Geometry check sheet. Reference: the model listing, model coordinates, mm. Give positions to 0.01 mm unless a question says otherwise; leave off trailing zeros. Loops run counter-clockwise (first coordinate to the right, second up) from the corner with the lowest first, then second, coordinate; pieces in that order, holes last. Notation, with made-up numbers: (-24.75, 66) - (16.25, 66) arc R20 cw to (16.25, 77) - close; hole circle Ø7 at (-14.5, -37.75). An arc over 180 degrees is marked (long way). Use a Markdown table: item, result. Add a question column.
1. Draft check along Y on faces 1 (the cylindrical face through (5.48, 1.67, -0.53)), 2 (the flat face through (0, -1, -1)), 3 (the conical face through (2.34, -0.02, 0.07)). Enter one of: pulls with the +Y half, pulls with the -Y half, needs draft (parallel to the pull), parting line crosses it, or undercut.
2. Cross-section at A-A on x = 1. Enter the section's corners in (y, z).
3. Material ranges on L1, parallel to Y at x = 0.5, z = 0.75; L2, parallel to X at y = -0.5, z = -2; L3, parallel to X at y = 3, z = 0, recorded low to high.
4. Cross-section at B-B on x = 5.75. Enter the section's corners in (y, z).
5. Depth check by flat-ended pin: P1, Ø1, axis at x = 7, z = 0.5, coming from the -Y side; P2, Ø1.5, axis at x = 6, z = -2, coming from the +Y side; P3, Ø1.5, axis at y = 2, z = 2.5, coming from the +X side. Enter the tip coordinate at first touch or a pass-through.
Autodesk Inventor part; units mm, degrees
ref_plane "Work Plane1" through (66.6877, 0, 0) normal (0, 0, -1) x (1, 0, 0)
ref_plane "YZ Plane" through (0, 0, 0) normal (1, 0, 0) x (0, 1, 0)
ref_plane "XZ Plane" through (0, 0, 0) normal (0, 1, 0) x (-1, 0, 0)
sketch "Sketch1" plane through (0, 0, 0) normal (0, 0, 1) x (1, 0, 0)
  line L0 (9.525, 0) -> (9.525, 1.7526)
  line L1 (9.525, 1.7526) -> (2.4638, 1.7526)
  line L2 (0, 3.3401) -> (0, 1.2192)
  line L3 (0, 1.2192) -> (1.6764, 1.2192)
  line L4 (1.6764, 1.2192) -> (2.3803, 0)
  line L5 (2.3803, 0) -> (9.525, 0)
  line L6 (0, 3.3401) -> (0.6376, 3.3401)
  line L7 (0.6376, 3.3401) -> (2.4638, 1.7526)
  line L8 (-1.905, 0) -> (11.43, 0)
  line L9 (0, -0.668) -> (0, 4.0081)
  dimension "d0" = 9.525
  dimension "d1" = 1.6764
  dimension "d2" = 3.5052
  dimension "d3" = 2.4638
  dimension "d4" = 41
  dimension "d5" = 2.4384
  dimension "d6" = 60
  dimension "d7" = 6.6802
revolve "Body" add sketch "Sketch1" angle 360 about axis through (2.3803, 0, 0) along (1, 0, 0) contours L5 L4 L3 L2 L6 L7 L1 L0
sketch "Sketch2" plane through (0, 0, 0) normal (-1, 0, 0) x (0, 0, 1)
  circle A0 centre (0, 0) radius 3.3401
  circle A1 centre (0, 0) radius 1.2192
  line L0 (0.9421, 0.2524) -> (1.1777, 0.3156)
  line L1 (0.9421, -0.2524) -> (1.1777, -0.3156)
  arc A2 (0.9421, -0.2524) -> (0.9421, 0.2524) centre (0, 0) ccw
  arc A3 (1.1777, -0.3156) -> (1.1777, 0.3156) centre (0, 0) ccw
  line L2 (0, -4.6761) -> (0, 4.6761)
  line L3 (-4.6761, 0) -> (4.6761, 0)
  line L4 (0.9421, 0.2524) -> (0, 0) construction
  line L5 (0, 0) -> (0.9421, -0.2524) construction
  line L6 (0.2524, 0.9421) -> (0.3156, 1.1777)
  line L7 (0.6897, 0.6897) -> (0.8621, 0.8621)
  arc A4 (0.6897, 0.6897) -> (0.2524, 0.9421) centre (0, 0) ccw
  arc A5 (0.8621, 0.8621) -> (0.3156, 1.1777) centre (0, 0) ccw
  line L8 (-0.6897, 0.6897) -> (-0.8621, 0.8621)
  line L9 (-0.2524, 0.9421) -> (-0.3156, 1.1777)
  arc A6 (-0.2524, 0.9421) -> (-0.6897, 0.6897) centre (0, 0) ccw
  arc A7 (-0.3156, 1.1777) -> (-0.8621, 0.8621) centre (0, 0) ccw
  line L10 (-0.9421, -0.2524) -> (-1.1777, -0.3156)
  line L11 (-0.9421, 0.2524) -> (-1.1777, 0.3156)
  arc A8 (-0.9421, 0.2524) -> (-0.9421, -0.2524) centre (0, 0) ccw
  arc A9 (-1.1777, 0.3156) -> (-1.1777, -0.3156) centre (0, 0) ccw
  line L12 (-0.2524, -0.9421) -> (-0.3156, -1.1777)
  line L13 (-0.6897, -0.6897) -> (-0.8621, -0.8621)
  arc A10 (-0.6897, -0.6897) -> (-0.2524, -0.9421) centre (0, 0) ccw
  arc A11 (-0.8621, -0.8621) -> (-0.3156, -1.1777) centre (0, 0) ccw
  line L14 (0.6897, -0.6897) -> (0.8621, -0.8621)
  line L15 (0.2524, -0.9421) -> (0.3156, -1.1777)
  arc A12 (0.2524, -0.9421) -> (0.6897, -0.6897) centre (0, 0) ccw
  arc A13 (0.3156, -1.1777) -> (0.8621, -0.8621) centre (0, 0) ccw
  dimension "d8" = 1.9507
  dimension "d9" = 2.4384
  dimension "d10" = 15
  dimension "d11" = 15
  dimension "d22" = 360
extrude "Slot" add sketch "Sketch2" against normal up to next contours L3 A2 L0 A1 | A1 L1 A2 L3 | L3 A8 L10 A1 | A1 L11 A8 L3 | A1 L7 A4 L6 | L9 A6 L8 A1 | A1 L13 A10 L12 | L15 A12 L14 A1
thread "Thread"
chamfer "Chamfer1" distance 0.4724 distance2 0.9449 1 edges at (9.525, -1.7526, 0) measured on face at (9.525, 0.5842, 0.7748)
ref_plane "Work Plane1" through (66.6877, 0, 0) normal (0, 0, -1) x (1, 0, 0)
equation "\"d0\" = NLG"
equation "\"d1\" = INTI"
equation "\"d2\" = GD"
equation "\"d3\" = KOH"
equation "\"d4\" = 0.5 * SEWI"
equation "\"d5\" = SW"
equation "\"d7\" = KOD"
equation "\"d8\" = 0.8 * SW"
equation "\"d9\" = SW"
equation "\"d15\" = GEL"
equation "\"d17\" = -0.5 * SPD + 0.5 * GD"
equation "\"d18\" = GUL"
equation "\"NLG\" = 9.525"
equation "\"SW\" = 2.4384"
equation "\"INTI\" = 1.6764"
equation "\"GEL\" = 5.07695"
equation "\"KOH\" = 2.4638"
equation "\"KOD\" = 6.6802"
equation "\"GUL\" = 0.94488"
equation "\"SPD\" = 2.56032"
equation "\"GD\" = NND"
equation "\"SEWI\" = 82deg"
equation "\"TOA\" = 30deg"
equation "\"GD1\" = SPD"
equation "\"EPV\" = 4.4794"
equation "\"THREADDIA\" = 3.5052"
equation "\"BDM\" = NND"
equation "\"NND\" = 3.5052"
equation "\"GAL\" = 1.9845"
equation "\"E0\" = 1.155 * SW"
properties part number "ANSI B18.3 - 6-32 UNC x 0.375, SSFCHCSI" material "Steel, Mild"
Values found:
| question | item | result |
|---|---|---|
| 1 | face 1 | parting line crosses it |
| 1 | face 2 | needs draft |
| 1 | face 3 | undercut |
| 2 | outline | circle Ø6.05 at (0, 0); hole (-1.18, -0.32) - (-0.94, -0.25) arc R0.97 ccw to (-0.69, -0.69) - (-0.86, -0.86) arc R1.22 ccw to (-0.32, -1.18) - (-0.25, -0.94) arc R0.98 ccw to (0.25, -0.94) - (0.32, -1.18) arc R1.22 ccw to (0.86, -0.86) - (0.69, -0.69) arc R0.98 ccw to (0.94, -0.25) - (1.18, -0.32) arc R1.22 ccw to (1.18, 0.32) - (0.94, 0.25) arc R0.97 ccw to (0.69, 0.69) - (0.86, 0.86) arc R1.22 ccw to (0.32, 1.18) - (0.25, 0.94) arc R0.98 ccw to (-0.25, 0.94) - (-0.32, 1.18) arc R1.22 ccw to (-0.86, 0.86) - (-0.69, 0.69) arc R0.98 ccw to (-0.94, 0.25) - (-1.18, 0.32) arc R1.22 ccw to start |
| 3 | L1 | y = -3.25 to -0.75, 0.75 to 3.25 |
| 3 | L2 | x = 0 to 2.11 |
| 3 | L3 | x = 0 to 1.03 |
| 4 | outline | circle Ø3.51 at (0, 0) |
| 5 | P1 | stops at y = -1.75 |
| 5 | P2 | stops at y = 1.23 |
| 5 | P3 | stops at x = 1.66 |
